```python
from build123d import *

# Parameters (mm, degrees)
SKETCH1_R            = 1.25
BOSS_EXTRUDE1_DEPTH  = 3
SKETCH2_W            = 18
SKETCH2_H            = 2.5
BOSS_EXTRUDE2_DEPTH  = 15
MOVE_START           = -15
MOVE_FACE1_DEPTH     = 18
M3_CLEARANCE_HOLE1_D = 3.4


# Read off the part's stored shape, not the designer's step: Move Face1
with BuildPart() as part:
    # Sketch1 → Boss-Extrude1 (new body)
    with BuildSketch(Plane.XY):
        with BuildLine():
            Line((24.479890084, 11.071980885), (-18.520109916, 49.071980885))
            ThreePointArc((-18.520109916, 49.071980885), (-24.871980885, 48.679890084), (-24.479890084, 42.328019115))
            Line((-24.479890084, 42.328019115), (-9, 28.64811625))
            Line((-9, 28.64811625), (-9, 0))
            Line((-9, 0), (9, 0))
            Line((9, 0), (9, 12.741139506))
            Line((9, 12.741139506), (18.520109916, 4.328019115))
            ThreePointArc((18.520109916, 4.328019115), (24.871980885, 4.720109916), (24.479890084, 11.071980885))
        make_face()
        with Locations((21.5, 7.7)):
            Circle(SKETCH1_R, mode=Mode.SUBTRACT)
        with Locations((-21.5, 45.7)):
            Circle(SKETCH1_R, mode=Mode.SUBTRACT)
    extrude(amount=BOSS_EXTRUDE1_DEPTH)

    # Sketch2 → Boss-Extrude2 (add)
    with BuildSketch(Plane(origin=(0, 0, 0), x_dir=(-1, 0, 0), z_dir=(0, 0, -1))):
        with Locations((0, 1.25)):
            Rectangle(SKETCH2_W, SKETCH2_H)
    extrude(amount=BOSS_EXTRUDE2_DEPTH)

    # Move Face1 outline → Move Face1 (cut)
    with BuildSketch(Plane.XY.offset(MOVE_START)):
        Polygon((-6.5, 26.438813925), (-9, 28.64811625), (-9, 0), (-6.5, 0), align=None)
    extrude(amount=MOVE_FACE1_DEPTH, mode=Mode.SUBTRACT)

    # M3 Clearance Hole1 (through all)
    with Locations(Plane(origin=(0, 2.5, 0), x_dir=(1, 0, 0), z_dir=(0, 1, 0))):
        with Locations((-2.285533906, 3.964466094), (4.785533906, 11.035533906)):
            Hole(M3_CLEARANCE_HOLE1_D / 2)


solid = part.part
```
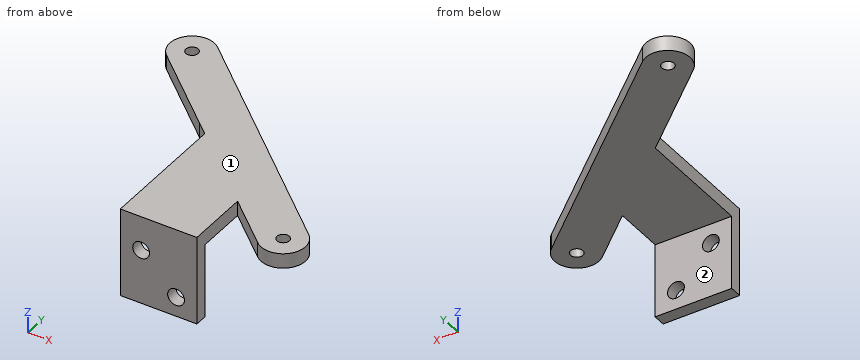
Design review of the part built by this model. Coordinates are the model's own, in mm. Face numbers are marked on the shaded views. A direction names the side the tool comes from. Give positions to 0.01 mm unless a question says otherwise; leave off trailing zeros. Order: outer loops, then holes, each group sorted by start corner. A loop starts at its lowest first (then second) coordinate and runs counter-clockwise, first axis right, second up. Notation, with made-up numbers: (-11.5, 31) -> (11.5, 31) arc R32 cw to (11.5, 65) -> close; hole circle Ø9 at (33, -10.75). An arc over 180 degrees is marked (long way). Write each question's results on one line, items separated by ' | '. Start each with the question number.
Q1. Add section D-D on x = 21.5. Give the boundary of the cut face in (y, z).
Q2. For pin 1 (1 mm diameter, centred on y = 40.5, z = 1, fed in from +X); pin 2 (3 mm diameter, centred on x = 21.5, y = 7.7, fed in from -Z); pin 3 (5 mm diameter, centred on x = -2, z = -5.5, fed in from +Y), all flat-tipped, find the tip position at first contact; note any pin that passes through.
Q3. Add section B-B on y = 45.7. Give the boundary of the cut face in (x, z), and give its area (3 significant figures).
Q4. Wall thickness on L1, parallel to Y at x = 7, z = -3.5; L2, parallel to Z at x = 8.5, y = 23; L3, parallel to X at y = 45, z = 1.25: over which ranges is each line inside the solid? List them lowest first. Write a range as from..to.
Q5. Add section A-A on x = 4.5. Give the boundary of the cut face in (y, z), and give its area (3 significant figures).
Q6. Machinability: for the marked faces 1 and 2, which of the approach directions +Z, -Z, +X, -X, +Y, -Y give a long, thin tool a straight path to every point of the face, cutting with its end or side? Answer none if there is none.
Q7. Add section C-C on y = 7.7. Give the boundary of the cut face in (x, z), and give its area (3 significant figures).
Found:
1) outline: (3.2, 0) -> (6.45, 0) -> (6.45, 3) -> (3.2, 3) -> close; (8.95, 0) -> (13.71, 0) -> (13.71, 3) -> (8.95, 3) -> close
2) pin 1: stops at x = -8.25 | pin 2: stops at z = 0 | pin 3: stops at y = 2.5
3) outline: (-26, 0) -> (-22.75, 0) -> (-22.75, 3) -> (-26, 3) -> close; (-20.25, 0) -> (-14.7, 0) -> (-14.7, 3) -> (-20.25, 3) -> close | area: 26.4 mm2
4) L1: y = 0..2.5 | L2: z = 0..3 | L3: x = -25.95..-22.54, -20.46..-13.91
5) outline: (0, -15) -> (2.5, -15) -> (2.5, -12.71) -> (0, -12.71) -> close; (0, -9.36) -> (2.5, -9.36) -> (2.5, 0) -> (28.73, 0) -> (28.73, 3) -> (0, 3) -> close | area: 115 mm2
6) face 1: +Z, +X, -X, +Y, -Y | face 2: -Z, +X, -X, +Y
7) outline: (-6.5, 0) -> (9, 0) -> (9, 3) -> (-6.5, 3) -> close; (14.7, 0) -> (20.25, 0) -> (20.25, 3) -> (14.7, 3) -> close; (22.75, 0) -> (26, 0) -> (26, 3) -> (22.75, 3) -> close | area: 72.9 mm2
